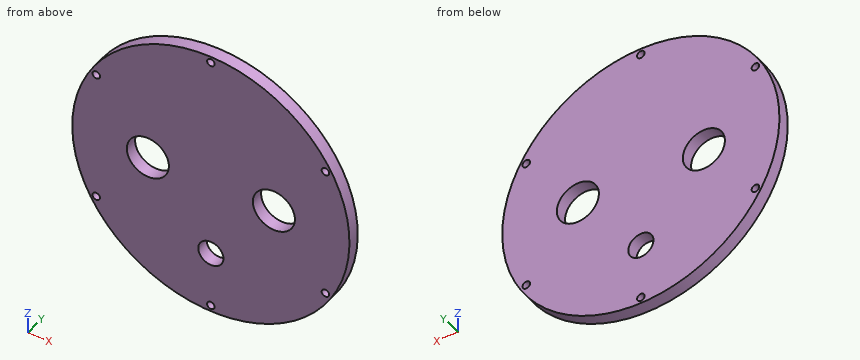
```python
from build123d import *

# Parameters (mm, degrees)
SKETCH_1_R          = 55
SKETCH_1_R_2        = 1.5
EXTRUDE_1_DEPTH     = 5
SKETCH_4_R          = 5
CUT_EXTRUDE_1_DEPTH = 10
SKETCH_5_R          = 8.35
CUT_EXTRUDE_2_DEPTH = 78.942286341


with BuildPart() as part:
    # 草图1 → 凸台-拉伸1 (new body)
    with BuildSketch(Plane(origin=(0, 0, 0), x_dir=(1, 0, 0), z_dir=(0, 1, 0))):
        with Locations(Location((0, 0, 0), (0, 0, 270))):
            Circle(SKETCH_1_R)
        with Locations(Location((0, 52.5, 0), (0, 0, 270))):
            Circle(SKETCH_1_R_2, mode=Mode.SUBTRACT)
        with Locations(Location((45.466333699, 26.25, 0), (0, 0, 270))):
            Circle(SKETCH_1_R_2, mode=Mode.SUBTRACT)
        with Locations(Location((45.466333699, -26.25, 0), (0, 0, 270))):
            Circle(SKETCH_1_R_2, mode=Mode.SUBTRACT)
        with Locations(Location((0, -52.5, 0), (0, 0, 270))):
            Circle(SKETCH_1_R_2, mode=Mode.SUBTRACT)
        with Locations(Location((-45.466333699, -26.25, 0), (0, 0, 270))):
            Circle(SKETCH_1_R_2, mode=Mode.SUBTRACT)
        with Locations(Location((-45.466333699, 26.25, 0), (0, 0, 270))):
            Circle(SKETCH_1_R_2, mode=Mode.SUBTRACT)
    extrude(amount=EXTRUDE_1_DEPTH)

    # 草图4 → 切除-拉伸1 (cut)
    with BuildSketch(Plane(origin=(0, 5, 0), x_dir=(1, 0, 0), z_dir=(0, 1, 0))):
        with Locations(Location((0, 30, 0), (0, 0, 270))):
            Circle(SKETCH_4_R)
    extrude(amount=-CUT_EXTRUDE_1_DEPTH, mode=Mode.SUBTRACT)

    # 草图5 → 切除-拉伸2 (cut, through all)
    with BuildSketch(Plane.XZ):
        with Locations(Location((-25, 0, 0), (0, 0, 270))):
            Circle(SKETCH_5_R)
        with Locations(Location((25, 0, 0), (0, 0, 270))):
            Circle(SKETCH_5_R)
    extrude(amount=-CUT_EXTRUDE_2_DEPTH, mode=Mode.SUBTRACT)


solid = part.part
```
The model under review builds one solid part; all positions refer to its coordinate system, in mm. Round coordinates to 2 decimals unless told otherwise and drop trailing zeros. Loops run counter-clockwise (first coordinate to the right, second up) from the corner with the lowest first, then second, coordinate; pieces in that order, holes last. Notation, with made-up numbers: (-8, 62.5) - (7, 62.5) arc R9 ccw to (7, 66.5) - close; hole circle Ø3 at (-11.75, 84.5). An arc over 180 degrees is marked (long way). Use a Markdown table: item, result. Add a question column.
Q1. Insertion check: pin 1 Ø1.5 at (y, z) = (3, -3.5) entering from -X; pin 2 Ø1.5 at (y, z) = (2.5, -21) entering from +X. Each pin has a flat end and moves straight along its axis. Give the tip position at first contact, or say it passes through.
Q2. Add section A-A (x = -31.5). State the section outline as (y, z) points, plus the area to 3 significant figures.
Q3. Add section D-D (x = 0). State the section outline as (y, z) points, plus the area to 3 significant figures.
Q4. Add section B-B (z = -52.5). State the section outline as (x, y) points.
Q5. For probe 1 along X at (y, z) = (1.3, -0.5); probe 2 along Z at (x, y) = (-1, 4.7); probe 3 along X at (y, z) = (4.05, -2), list the stretches that pass through material, from the lowest coordinate up.
Q6. Add section C-C (y = 3.45). State how many separate pieces and enclosed holes the cut face has, plus the area to 3 significant figures.
Worked answers:
| question | item | result |
|---|---|---|
| 1 | pin 1 | x = -54.93 |
| 1 | pin 2 | x = 51.14 |
| 2 | outline | (0, -45.09) - (5, -45.09) - (5, -5.24) - (0, -5.24) - close; (0, 5.24) - (5, 5.24) - (5, 45.09) - (0, 45.09) - close |
| 2 | area | 398 mm² |
| 3 | outline | (0, -55) - (5, -55) - (5, -54) - (0, -54) - close; (0, -51) - (5, -51) - (5, -35) - (0, -35) - close; (0, -25) - (5, -25) - (5, 51) - (0, 51) - close; (0, 54) - (5, 54) - (5, 55) - (0, 55) - close |
| 3 | area | 470 mm² |
| 4 | outline | (-16.39, 0) - (-1.5, 0) - (-1.5, 5) - (-16.39, 5) - close; (1.5, 0) - (16.39, 0) - (16.39, 5) - (1.5, 5) - close |
| 5 | probe 1 | -55 to -33.34, -16.66 to 16.66, 33.34 to 55 |
| 5 | probe 2 | -54.99 to -53.62, -51.38 to -34.9, -25.1 to 51.38, 53.62 to 54.99 |
| 5 | probe 3 | -54.96 to -33.11, -16.89 to 16.89, 33.11 to 54.96 |
| 6 | separate pieces | 1 |
| 6 | enclosed holes | 9 |
| 6 | area | 8,940 mm² |
